from build123d import *

# Parameters (mm, degrees)
BOSS_EXTRUDE1_DEPTH = 3.175
BOSS_EXTRUDE2_DEPTH = 3.175
FILLET1_R           = 1.5875
BOSS_EXTRUDE3_DEPTH = 3.175
FILLET2_R           = 1.5875


with BuildPart() as part:
    # Sketch1 → Boss-Extrude1 (new body)
    with BuildSketch(Plane(origin=(0, 0, 0), x_dir=(0, 0, -1), z_dir=(1, 0, 0))):
        Polygon((-123.554053147, -17.526), (-66.404053147, -103.885992991), (-66.404053147, -118.573420749), (-98.706493282, -118.573420749), (-123.554053147, -81.026), (-142.875, -81.026), (-142.875, -17.526), align=None)
        with BuildLine():
            Line((-132.324466277, -23.876), (-129.904053147, -23.876))
            ThreePointArc((-129.904053147, -23.876), (-110.14576301, -72.890584378), (-72.754053147, -110.235992991))
            Line((-72.754053147, -110.235992991), (-74.065724778, -112.223420749))
            ThreePointArc((-74.065724778, -112.223420749), (-112.252146658, -74.022181286), (-132.324466277, -23.876))
        make_face(mode=Mode.SUBTRACT)
    extrude(amount=BOSS_EXTRUDE1_DEPTH)

    # Sketch2 → Boss-Extrude2 (add)
    with BuildSketch(Plane(origin=(0, -17.526, 0), x_dir=(1, 0, 0), z_dir=(0, 1, 0))):
        Polygon((0, -123.554053147), (3.175, -123.554053147), (3.175, -174.625), (-15.875, -174.625), (-15.875, -142.875), align=None)
    extrude(amount=BOSS_EXTRUDE2_DEPTH)

    # Fillet1
    # the kernel refuses this fillet: 1.5875 mm, written as the material it adds along each edge
    with BuildSketch(Plane(origin=(0, -17.526, 123.554053147), x_dir=(0, -0.8339321851132224, -0.5518669319974573), z_dir=(1, 0, 0))) as fillet1_piece_1:
        with BuildLine():
            CenterArc((FILLET1_R * 0.300920032091, FILLET1_R), FILLET1_R, 236.504813186, 33.495186814)
            Line((-FILLET1_R * 0.250946899906, FILLET1_R * 0.166067814887), (0, 0))
            Line((0, 0), (FILLET1_R * 0.300920032091, 0))
        make_face()
    extrude(amount=3.175)
    # the kernel refuses this fillet: 1.5875 mm, written as the material it takes off along each edge
    with BuildSketch(Plane(origin=(-18.394522192, -14.351, 145.941428621), x_dir=(0.7726434320880118, 0, 0.6348402372654539), z_dir=(0.634840237265454, 0, -0.7726434320880119))) as fillet1_2_piece_1:
        with BuildLine():
            CenterArc((FILLET1_R, FILLET1_R), FILLET1_R, 180, 90)
            Line((0, FILLET1_R), (0, 0))
            Line((0, 0), (FILLET1_R, 0))
        make_face()
    extrude(amount=32.943791454, mode=Mode.SUBTRACT)
    with BuildSketch(Plane(origin=(-15.875, -14.351, 178.59375), x_dir=(1, 0, 0), z_dir=(0, 0, -1))) as fillet1_2_piece_2:
        with BuildLine():
            CenterArc((FILLET1_R, FILLET1_R), FILLET1_R, 180, 90)
            Line((0, FILLET1_R), (0, 0))
            Line((0, 0), (FILLET1_R, 0))
        make_face()
    extrude(amount=39.6875, mode=Mode.SUBTRACT)
    with BuildSketch(Plane(origin=(7.14375, -14.351, 174.625), x_dir=(0, -1, 0), z_dir=(-1, 0, 0))) as fillet1_2_piece_3:
        with BuildLine():
            CenterArc((FILLET1_R, -FILLET1_R), FILLET1_R, 90, 90)
            Line((0, -FILLET1_R), (0, 0))
            Line((0, 0), (FILLET1_R, 0))
        make_face()
    extrude(amount=26.9875, mode=Mode.SUBTRACT)
    with BuildSketch(Plane(origin=(3.175, -14.351, 119.585303147), x_dir=(0, -1, 0), z_dir=(0, 0, 1))) as fillet1_2_piece_4:
        with BuildLine():
            CenterArc((FILLET1_R, -FILLET1_R), FILLET1_R, 90, 90)
            Line((0, -FILLET1_R), (0, 0))
            Line((0, 0), (FILLET1_R, 0))
        make_face()
    extrude(amount=59.008446853, mode=Mode.SUBTRACT)
    with BuildSketch(Plane(origin=(-3.96875, -14.351, 123.554053147), x_dir=(0, 0, 1), z_dir=(1, 0, 0))) as fillet1_2_piece_5:
        with BuildLine():
            CenterArc((FILLET1_R, FILLET1_R), FILLET1_R, 180, 90)
            Line((0, FILLET1_R), (0, 0))
            Line((0, 0), (FILLET1_R, 0))
        make_face()
    extrude(amount=11.1125, mode=Mode.SUBTRACT)

    # Sketch4 → Boss-Extrude3 (add)
    with BuildSketch(Plane.XZ.offset(81.026)):
        Polygon((3.175, 123.554053147), (3.175, 174.625), (-15.875, 174.625), (-15.875, 142.875), (0, 123.554053147), align=None)
    extrude(amount=BOSS_EXTRUDE3_DEPTH)

    # Fillet2
    fillet2_edges = [part.edges().sort_by_distance(p)[0] for p in [
        (1.5875, -84.201, 123.554053147),
        (3.175, -84.201, 149.089526573),
        (-6.35, -84.201, 174.625),
        (-15.875, -84.201, 158.75),
        (-7.9375, -84.201, 133.214526573),
    ]]
    fillet(fillet2_edges, radius=FILLET2_R)


solid = part.part
Verification items for the finished model (mm, model axes). A direction names the side the tool comes from. Round coordinates to 2 decimals unless told otherwise and drop trailing zeros. Write each loop counter-clockwise with the first axis right and the second up, starting at its lowest first coordinate (ties: lowest second). Pieces come first, ordered by that corner, then holes.
(1) Section check B-B (y = -109). Enter the section's corners in (x, z) (3 decimals), plus the area to 3 significant figures.
Returned:
outline: (0, 66.404) - (3.175, 66.404) - (3.175, 74.593) - (0, 74.593) - close; (0, 78.733) - (3.175, 78.733) - (3.175, 105.042) - (0, 105.042) - close
area: 110 mm2
(2) Section check C-C (y = -47.5). Enter the section's corners in (x, z) (3 decimals), plus the area to 3 significant figures.
Returned:
outline: (0, 103.718) - (3.175, 103.718) - (3.175, 123.243) - (0, 123.243) - close; (0, 125.792) - (3.175, 125.792) - (3.175, 142.875) - (0, 142.875) - close
area: 116 mm2
(3) Mould release check, pull along Y, two halves, no side actions. Record for faces 6 (the flat face through (2, -100, 111)), 7 (the flat face through (2, -111, 66.404)), 8 (the flat face through (2, -50, 142.875)): pulls with the +Y half, pulls with the -Y half, needs draft (parallel to the pull), parting line crosses it, or undercut.
Returned:
face 6: pulls with the -Y half
face 7: needs draft
face 8: undercut
(4) Section check A-A (z = 152.5). Enter the section's corners in (x, y) (1 decimal), plus the area to 3 significant figures.
Returned:
outline: (-15.9, -82.6) arc R1.6 ccw to (-14.3, -84.2) - (1.6, -84.2) arc R1.6 ccw to (3.2, -82.6) - (3.2, -81) - (-15.9, -81) - close; (-15.9, -17.5) - (3.2, -17.5) - (3.2, -15.9) arc R1.6 ccw to (1.6, -14.4) - (-14.3, -14.4) arc R1.6 ccw to (-15.9, -15.9) - close
area: 119 mm2
(5) Material ranges on line 1 (Y direction, x = 1.75, z = 152); line 2 (Y direction, x = 0.5, z = 92.5); line 3 (X direction, y = -72.5, z = 126) (3 decimals), recorded low to high.
Returned:
line 1: y = -84.19 to -81.03, -17.53 to -14.36
line 2: y = -118.57 to -97.59, -94.28 to -64.45
line 3: x = 0 to 3.175
(6) Depth check by flat-ended pin: pin 1 Ø0.5 at (x, y) = (1, -82) entering from -Z; pin 2 Ø8 at (x, z) = (-3, 144.5) entering from -Y; pin 3 Ø2.5 at (x, y) = (2, -53.5) entering from +Z (3 decimals). Enter the tip coordinate at first touch or a pass-through.
Returned:
pin 1: stops at z = 80.72
pin 2: stops at y = -84.2
pin 3: stops at z = 142.875
(7) Access from +Z, -Z, +X, -X, +Y, -Y to the whole of each face (thin tool, end or side, straight path). Record for faces 1 (the flat face through (-8.05, -81.81, 133.35)), 2 (the cylindrical face through (-7.7, -14.83, 133.64)), 3 (the flat face through (-6, -17.526, 154)), 4 (the cylindrical face through (1.565, -72.268, 110.555)), 5 (the flat face through (-6, -84.201, 155)).
Returned:
face 1: -Z, -X, +Y, -Y
face 2: -Z, -X, +Y
face 3: +Z, -X
face 4: +X, -X
face 5: +Z, +X, -X, -Y
